from build123d import *
from build123d.topology import SkipClean

# Parameters (mm, degrees)
SKETCH10_R              = 10
BOSS_EXTRUDE1_DEPTH     = 5
CUT_EXTRUDE3_DEPTH      = 45
CUT_EXTRUDE3_DEPTH_BACK = 20
SKETCH12_W              = 60
SKETCH12_H              = 3
CUT_EXTRUDE4_DEPTH      = 28


with BuildPart() as part:
    # Sketch1 → Revolve1 (revolve)
    with BuildSketch(Plane.XY):
        with BuildLine():
            Line((20.9, 0), (23.871591838, 0))
            Line((23.871591838, 0), (23.871591838, 4))
            Line((23.871591838, 4), (22.9, 4.236662843))
            Line((22.9, 4.236662843), (22.9, 11.404308102))
            ThreePointArc((22.9, 11.404308102), (23.83692213, 15.63049072), (26.472123903, 19.064752533))
            Line((26.472123903, 19.064752533), (26.988320528, 19.497892931))
            ThreePointArc((26.988320528, 19.497892931), (29.623522302, 22.932154745), (30.560444431, 27.158337362))
            Line((30.560444431, 27.158337362), (30.560444431, 50))
            ThreePointArc((30.560444431, 50), (29.388871556, 52.828427125), (26.560444431, 54))
            Line((26.560444431, 54), (2.764914955, 54))
            Line((2.764914955, 54), (2.764914955, 15))
            Line((2.764914955, 15), (19.9, 15))
            ThreePointArc((19.9, 15), (20.607106781, 14.707106781), (20.9, 14))
            Line((20.9, 14), (20.9, 0))
        make_face()
    revolve(axis=Axis((2.764914955, 7.821821657, 0), (0, 1, 0)))

    # Sketch10 → Boss-Extrude1 (add)
    with SkipClean():  # the faces are left unmerged after this step: merging them gives an invalid solid
        with BuildSketch(Plane.XY.offset(27.795529476)):
            with Locations((3.346345887, 38.658337362)):
                Circle(SKETCH10_R)
        extrude(amount=-BOSS_EXTRUDE1_DEPTH)

    # Sketch11 → Cut-Extrude3 (cut, two sides: drawn at the far end of the back side and taken through both)
    with SkipClean():  # the faces are left unmerged after this step: merging them gives an invalid solid
        with BuildSketch(Plane(origin=(0, 17, 0), x_dir=(1, 0, 0), z_dir=(0, 1, 0)).offset(-CUT_EXTRUDE3_DEPTH_BACK)):
            with BuildLine():
                Line((-14.735085045, 0), (20.264914955, 0))
                ThreePointArc((20.264914955, 0), (2.764914955, 17.5), (-14.735085045, 0))
            make_face()
        extrude(amount=CUT_EXTRUDE3_DEPTH + CUT_EXTRUDE3_DEPTH_BACK, mode=Mode.SUBTRACT)

    # Sketch12 → Cut-Extrude4 (cut)
    with SkipClean():  # the faces are left unmerged after this step: merging them gives an invalid solid
        with BuildSketch(Plane.XY.offset(27.795529476)):
            with Locations((3.002856973, 51)):
                Rectangle(SKETCH12_W, SKETCH12_H)
        extrude(amount=-CUT_EXTRUDE4_DEPTH, mode=Mode.SUBTRACT)


solid = part.part
Input: part model. Units: mm. Frame: model coordinates. A direction names the side the tool comes from. Coordinates: 2 decimals unless noted, no trailing zeros. Order: outer loops, then holes, each group sorted by start corner. A loop starts at its lowest first (then second) coordinate and runs counter-clockwise, first axis right, second up. Notation, with made-up numbers: M 76.5,11.5 L 112.5,11.5 A22 cw 112.5,44.5 Z; hole C -25,70 d10. An arc over 180 degrees is marked long. Answer as CSV lines item,"result".
1. Pull-direction query (X, two-part tool) for faces 1 (the flat face through (-20, 51, -0.204)), 2 (the cylindrical face through (3.15, 34.192, -17.496)), 3 (the cylindrical face through (-13.214, 7.871, 12.252)), 4 (the cylindrical face through (12.5, 6.9, -15.3)); classes: released by +X, released by -X, zero draft, split by the parting line, or undercut.
Reported:
face 1,"zero draft"
face 2,"undercut"
face 3,"split by the parting line"
face 4,"undercut"
2. Section A-A (y = 44). Return the cut outline in (x, z), then the cut area to 3 significant figures.
Reported:
outline,"M -5.11,26.66 A27.8 ccw long 11.8,26.29 L 11.8,27.8 L -5.11,27.8 Z; hole M -14.74,0 A17.5 ccw 20.26,0 Z"
area,"1,950 mm2"
3. Material intervals for line 1 (Y direction, x = -5.5, z = 12.5); line 2 (X direction, y = 9.75, z = 0); line 3 (X direction, y = 3.5, z = 0), sorted ascending. Write a range as from..to.
Reported:
line 1,"15..49.5, 52.5..54"
line 2,"-17.37..-15.37, 20.9..22.9"
line 3,"-18.34..-15.37, 20.9..23.87"
4. First-contact query: P1, Ø1.5, axis at x = 23, y = 51, coming from the +Z side; P2, Ø2, axis at x = 12.5, z = 10.5, coming from the -Y side; P3, Ø8, axis at y = 37, z = 8, coming from the -X side. Flat tips, straight axial feed; report the tip coordinate or a pass-through.
Reported:
P1,"z = -0.2"
P2,"y = 15"
P3,"x = -24.74"
5. Access query for faces 5 (the flat face through (2, 52.5, 11)), 6 (the flat face through (3, 53, 0)), 7 (the flat face through (3, 15, 7)). Directions: +Z, -Z, +X, -X, +Y, -Y. A direction counts if a zero-diameter tool reaches every point of the face in a straight line with its end or side. Return the directions, or none.
Reported:
face 5,"+Z, +X, -X"
face 6,"+Y, -Y"
face 7,"-Y"
